The listing builds one solid part. Answer for the finished solid, in the listing's coordinates (mm). A direction names the side the tool comes from. Coordinates: 2 decimals unless noted, no trailing zeros. Order: outer loops, then holes, each group sorted by start corner. A loop starts at its lowest first (then second) coordinate and runs counter-clockwise, first axis right, second up. Notation, with made-up numbers: (-35.75, 3.5) -> (-5.75, 3.5) arc R25 cw to (-5.75, 30.5) -> close; hole circle Ø1 at (39.25, 11). An arc over 180 degrees is marked (long way). Return JSON: item names as keys, results as strings.
from build123d import *

# Parameters (mm, degrees)
F0_R          = 32.5
F1_DEPTH      = 50
F2_DEPTH      = 12
F4_DEPTH      = 6
F4_DEPTH_BACK = 6


with BuildPart() as f1:
    # F0 (on Top) → F1 (new body)
    with BuildSketch(Plane.XY):
        with BuildLine():
            ThreePointArc((82.5, 0), (54.860679775, 44.72135955), (2.5, 40))
            ThreePointArc((2.5, 40), (-17.5, 0), (2.5, -40))
            ThreePointArc((2.5, -40), (54.860679775, -44.72135955), (82.5, 0))
        make_face()
        with Locations((32.5, 0)):
            Circle(F0_R, mode=Mode.SUBTRACT)
    extrude(amount=F1_DEPTH)

    # F0 (on Top) → F2 (join)
    with BuildSketch(Plane.XY):
        with BuildLine():
            Line((2.5, 40), (-80, 40))
            Line((-80, 40), (-80, -40))
            Line((-80, -40), (2.5, -40))
            ThreePointArc((2.5, -40), (-17.5, 0), (2.5, 40))
        make_face()
        with BuildLine():
            ThreePointArc((82.5, 0), (54.860679775, 44.72135955), (2.5, 40))
            ThreePointArc((2.5, 40), (-17.5, 0), (2.5, -40))
            ThreePointArc((2.5, -40), (54.860679775, -44.72135955), (82.5, 0))
        make_face()
        with Locations((32.5, 0)):
            Circle(F0_R, mode=Mode.SUBTRACT)
    extrude(amount=F2_DEPTH)

    # F3 (on Front) → F4 (join, two sides)
    with BuildSketch(Plane.XZ) as f4_sk:
        Polygon((-15.4150407761, 46.4158691466), (-67.7281171784, 10.5064402626), (-15.4150407761, 10.5064402626), align=None)
    extrude(amount=-F4_DEPTH)
    extrude(f4_sk.sketch, amount=F4_DEPTH_BACK)


solid = f1.part
1. Each of these flat-tipped pins is pushed along its axis until it touches: pin 1 Ø1.5 at (y, z) = (29, 31.5) entering from -X; pin 2 Ø1.5 at (y, z) = (32.5, 39) entering from +X; pin 3 Ø6 at (x, y) = (61, -0.5) entering from +Z; pin 4 Ø8 at (x, z) = (-16.5, 34) entering from -Y. Where does it stop, or does it pass through?
Answer block:
{"pin 1": "stops at x = -8.75", "pin 2": "stops at x = 71.13", "pin 3": "passes through", "pin 4": "stops at y = -21.79"}
2. Determine the mould class of faces 1 (the face through (63.5, 9.76, 24.65)), 2 (the face through (81.645, 9.206, 24.65)), 3 (the face through (-38, 40, 6)) for opening direction Y: pulls with the +Y half, pulls with the -Y half, needs draft (parallel to the pull), parting line crosses it, or undercut.
Answer block:
{"face 1": "undercut", "face 2": "parting line crosses it", "face 3": "pulls with the +Y half"}
3. The part is cut by section A-A on x = 32.5. Give the vertices of the cut face in (y, z), and give its area (3 significant figures).
Answer block:
{"outline": "(-50, 0) -> (-32.5, 0) -> (-32.5, 50) -> (-50, 50) -> close; (32.5, 0) -> (50, 0) -> (50, 50) -> (32.5, 50) -> close", "area": "1,750 mm2"}
4. The part is cut by section C-C on z = 5. Give the vertices of the cut face in (x, y).
Answer block:
{"outline": "(-80, -40) -> (2.5, -40) arc R50 ccw (long way) to (2.5, 40) -> (-80, 40) -> close; hole circle Ø65 at (32.5, 0)"}
5. Consider line 1 (Y direction, x = 32.5, z = 14); line 2 (X direction, y = 4, z = 23); line 3 (X direction, y = 26, z = 37.5). Determine where each line is inside the solid, lowest interval first. Write a range as from..to.
Answer block:
{"line 1": "y = -50..-32.5, 32.5..50", "line 2": "x = -49.53..0.25, 64.75..82.34", "line 3": "x = -10.21..13, 52..75.21"}
6. The part is cut by section D-D on x = 14.5. Give the vertices of the cut face in (y, z).
Answer block:
{"outline": "(-46.65, 0) -> (-27.06, 0) -> (-27.06, 50) -> (-46.65, 50) -> close; (27.06, 0) -> (46.65, 0) -> (46.65, 50) -> (27.06, 50) -> close"}
7. For faces 4 (the face through (-31, -6, 21)), 5 (the face through (-39, -40, 6)), 6 (the face through (-31, 6, 21)), 7 (the face through (-48, 9, 12)), 8 (the face through (32, -33, 50)), determine the directions among +Z, -Z, +X, -X, +Y, -Y from which every point of the face is accessible in a straight line to the end or side of a thin tool.
Answer block:
{"face 4": "+Z, -X, -Y", "face 5": "+Z, -Z, -X, -Y", "face 6": "+Z, -X, +Y", "face 7": "+Z, -X", "face 8": "+Z, +X, -X, +Y, -Y"}
8. The part is cut by section B-B on y = 0. Give the vertices of the cut face in (x, z), and give its area (3 significant figures).
Answer block:
{"outline": "(-80, 0) -> (0, 0) -> (0, 50) -> (-17.5, 50) -> (-17.5, 44.98) -> (-65.55, 12) -> (-80, 12) -> close; (65, 0) -> (82.5, 0) -> (82.5, 50) -> (65, 50) -> close", "area": "3,290 mm2"}
